Here's how the part is built. I have some questions about the finished solid (model axes, mm). A direction names the side the tool comes from. Round coordinates to 2 decimals unless told otherwise and drop trailing zeros. Loops run counter-clockwise (first coordinate to the right, second up) from the corner with the lowest first, then second, coordinate; pieces in that order, holes last. Notation, with made-up numbers: (51.5, -5.75) - (81.5, -5.75) arc R11 cw to (81.5, 15.25) - close; hole circle Ø8 at (84, -13). An arc over 180 degrees is marked (long way). Answer as a JSON object with one key per item and string values. Group by question number.
1) I want a section at D-D, the plane x = -15.5. Please give me the cut outline in (y, z), then the cut area to 3 significant figures.
2) Will these pins go through, and if not, where does the flat tip stop? P1, Ø1, axis at y = 11.5, z = 20, coming from the +X side; P2, Ø2.5, axis at y = 15.5, z = 20.5, coming from the -X side; P3, Ø2, axis at x = -4, y = 6.5, coming from the -Z side; P4, Ø2, axis at x = -29, y = 14.5, coming from the +Z side.
3) I want a section at C-C, the plane y = 12.75. Please give me the cut outline in (x, z).
4) I want a section at B-B, the plane z = 6. Please give me the cut outline in (x, y).
5) I want a section at A-A, the plane y = 8.25. Please give me the cut outline in (x, z).
6) If we mould it in two halves opening along Z, with no side actions, what happens to faces 6 (the face through (-30, 12, 18.27)), 7 (the face through (-10, 13, 50.161)), 8 (the face through (-32.259, 12, 20))? For each: pulls with the +Z half, pulls with the -Z half, needs draft (parallel to the pull), parting line crosses it, or undercut.
7) If I drill on line 1 along Z through (x, y) = (-30.5, 16.5); line 2 along X through (y, z) = (14, 21.5); line 3 along Y through (x, z) = (-21, 50), over which ranges is the centre line in solid material (lowest first)? Write a range as [from, to].
8) Which directions (+Z, -Z, +X, -X, +Y, -Y) give clear straight access to the entire face, cutting with the end or side of a thin tool? Please do faces 1 (the face through (-22.238, 3, 5)), 2 (the face through (-9.107, 12, 53)), 3 (the face through (-25.221, 3, 6)), 4 (the face through (-30.794, 15, 21)), 5 (the face through (0, 2, 37)).
from build123d import *

# Parameters (mm, degrees)
AUFSATZ_LINEAR_AUSTRAGEN1_DEPTH = 5
AUFSATZ_LINEAR_AUSTRAGEN2_DEPTH = 5
SKIZZE5_R                       = 3
AUFSATZ_LINEAR_AUSTRAGEN3_DEPTH = 5
SKIZZE6_R                       = 1
SCHNITT_LINEAR_AUSTRAGEN3_DEPTH = 5
AUFSATZ_LINEAR_AUSTRAGEN4_DEPTH = 15
SKIZZE8_W                       = 20
SKIZZE8_H                       = 34
SCHNITT_LINEAR_AUSTRAGEN4_DEPTH = 15
SKIZZE9_W                       = 15.731932776
SKIZZE9_H                       = 1.345677625
SKIZZE9_W_2                     = 1.464910579
SKIZZE9_H_2                     = 28.562069045
SKIZZE9_H_3                     = 1.21563576
SKIZZE9_W_3                     = 1.686857954
SCHNITT_LINEAR_AUSTRAGEN5_DEPTH = 15
AUFSATZ_LINEAR_AUSTRAGEN5_DEPTH = 5


with BuildPart() as part:
    # Skizze1 → Aufsatz-Linear austragen1 (new body)
    with BuildSketch(Plane(origin=(0, 0, 0), x_dir=(1, 0, 0), z_dir=(0, 1, 0))):
        with BuildLine():
            Line((0, 0), (0, -75))
            ThreePointArc((0, -75), (-37.5, -37.5), (0, 0))
        make_face()
    extrude(amount=AUFSATZ_LINEAR_AUSTRAGEN1_DEPTH)

    # Skizze4 → Aufsatz-Linear austragen2 (add)
    with BuildSketch(Plane(origin=(0, 5, 0), x_dir=(1, 0, 0), z_dir=(0, 1, 0))):
        Polygon((-22.238082181, -7.305336549), (-22.238082181, 0.251909769), (-25.220656299, 0.251909769), (-25.220656299, -9.748090231), (-22.238082181, -9.748090231), align=None)
        Polygon((-22.238082181, -67.694663451), (-22.238082181, -75.251909769), (-25.220656299, -75.251909769), (-25.220656299, -65.251909769), (-22.238082181, -65.251909769), align=None)
    extrude(amount=-AUFSATZ_LINEAR_AUSTRAGEN2_DEPTH)

    # Skizze5 → Aufsatz-Linear austragen3 (add)
    with BuildSketch(Plane(origin=(0, 5, 0), x_dir=(1, 0, 0), z_dir=(0, 1, 0))):
        with Locations((-23.72936924, 0.251909769)):
            Circle(SKIZZE5_R)
        with Locations((-23.72936924, -75.251909769)):
            Circle(SKIZZE5_R)
    extrude(amount=-AUFSATZ_LINEAR_AUSTRAGEN3_DEPTH)

    # Skizze6 → Schnitt-Linear austragen3 (cut)
    with BuildSketch(Plane(origin=(0, 5, 0), x_dir=(1, 0, 0), z_dir=(0, 1, 0))):
        with Locations((-23.72936924, 0)):
            Circle(SKIZZE6_R)
        with Locations((-23.72936924, -75)):
            Circle(SKIZZE6_R)
    extrude(amount=-SCHNITT_LINEAR_AUSTRAGEN3_DEPTH, mode=Mode.SUBTRACT)

    # Skizze7 → Aufsatz-Linear austragen4 (add)
    with BuildSketch(Plane(origin=(0, 5, 0), x_dir=(1, 0, 0), z_dir=(0, 1, 0))):
        Polygon((-32.258719726, -18.830892905), (-32.258719726, -54.830892905), (-9.106951193, -54.830892905), (-9.106951193, -18.26957952), (-31.844703161, -18.26957952), align=None)
    extrude(amount=AUFSATZ_LINEAR_AUSTRAGEN4_DEPTH)

    # Skizze8 → Schnitt-Linear austragen4 (cut)
    with BuildSketch(Plane(origin=(0, 20, 0), x_dir=(1, 0, 0), z_dir=(0, 1, 0))):
        with Locations((-20.793809147, -36.48521528)):
            Rectangle(SKIZZE8_W, SKIZZE8_H)
    extrude(amount=-SCHNITT_LINEAR_AUSTRAGEN4_DEPTH, mode=Mode.SUBTRACT)

    # Skizze9 → Schnitt-Linear austragen5 (cut)
    with BuildSketch(Plane(origin=(0, 20, 0), x_dir=(1, 0, 0), z_dir=(0, 1, 0))):
        with Locations((-20.328643091, -54.158054093)):
            Rectangle(SKIZZE9_W, SKIZZE9_H)
        with Locations((-31.526264436, -35.879751076)):
            Rectangle(SKIZZE9_W_2, SKIZZE9_H_2)
        with Locations((-20.328643091, -18.8773974)):
            Rectangle(SKIZZE9_W, SKIZZE9_H_3)
        with Locations((-9.95038017, -35.879751076)):
            Rectangle(SKIZZE9_W_3, SKIZZE9_H_2)
    extrude(amount=-SCHNITT_LINEAR_AUSTRAGEN5_DEPTH, mode=Mode.SUBTRACT)

    # Skizze10 → Aufsatz-Linear austragen5 (add)
    with BuildSketch(Plane(origin=(0, 5, 0), x_dir=(1, 0, 0), z_dir=(0, 1, 0))):
        Polygon((-28.194609479, -53.48521528), (-30.793809147, -50.234762972), (-30.793809147, -53.48521528), align=None)
        Polygon((-30.793809147, -21.598716553), (-30.793809147, -19.48521528), (-28.194609479, -19.48521528), align=None)
        Polygon((-12.462676703, -19.48521528), (-10.793809147, -19.48521528), (-10.793809147, -21.598716553), align=None)
        Polygon((-12.462676703, -53.48521528), (-10.793809147, -53.48521528), (-10.793809147, -50.234762972), align=None)
    extrude(amount=AUFSATZ_LINEAR_AUSTRAGEN5_DEPTH)


solid = part.part
Outcome:
{
 "1": {"outline": "(0, 3.35) - (5, 3.35) - (5, 71.65) - (0, 71.65) - close", "area": "341 mm^2"},
 "2": {"P1": "x = -9.11", "P2": "x = -32.26", "P3": "through", "P4": "z = 54.83"},
 "3": {"outline": "(-32.26, 18.83) - (-31.84, 18.27) - (-28.19, 18.27) - (-28.19, 19.49) - (-30.79, 19.49) - (-30.79, 21.6) - (-32.26, 21.6) - close; (-32.26, 50.16) - (-30.79, 50.16) - (-30.79, 53.49) - (-28.19, 53.49) - (-28.19, 54.83) - (-32.26, 54.83) - close; (-12.46, 18.27) - (-9.11, 18.27) - (-9.11, 21.6) - (-10.79, 21.6) - (-10.79, 19.49) - (-12.46, 19.49) - close; (-12.46, 53.49) - (-10.79, 53.49) - (-10.79, 50.16) - (-9.11, 50.16) - (-9.11, 54.83) - (-12.46, 54.83) - close"},
 "4": {"outline": "(-25.22, 0) - (-22.24, 0) - (-22.24, 5) - (-25.22, 5) - close; (-20.35, 0) - (0, 0) - (0, 5) - (-20.35, 5) - close"},
 "5": {"outline": "(-32.26, 18.83) - (-31.84, 18.27) - (-28.19, 18.27) - (-28.19, 19.49) - (-30.79, 21.6) - (-32.26, 21.6) - close; (-32.26, 50.16) - (-30.79, 50.16) - (-30.79, 50.23) - (-28.19, 53.49) - (-28.19, 54.83) - (-32.26, 54.83) - close; (-12.46, 18.27) - (-9.11, 18.27) - (-9.11, 21.6) - (-10.79, 21.6) - (-12.46, 19.49) - close; (-12.46, 53.49) - (-10.79, 50.23) - (-10.79, 50.16) - (-9.11, 50.16) - (-9.11, 54.83) - (-12.46, 54.83) - close"},
 "6": {"face 6": "pulls with the -Z half", "face 7": "undercut", "face 8": "needs draft"},
 "7": {"line 1": "[18.27, 19.49], [53.49, 54.83]", "line 2": "[-32.26, -30.79], [-10.79, -9.11]", "line 3": "[0, 5]"},
 "8": {"face 1": "+Y, -Y", "face 2": "+Z, -Z, +X, +Y", "face 3": "-X, +Y, -Y", "face 4": "+Y", "face 5": "+Z, -Z, +X, +Y, -Y"}
}
